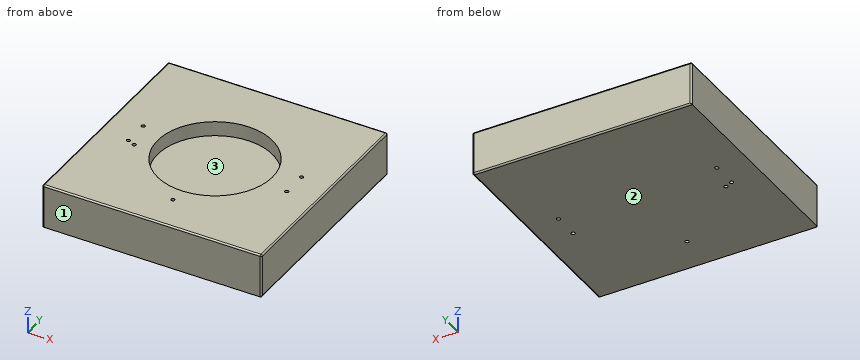
```python
from build123d import *

# Parameters (mm, degrees)
SKETCH1_W                   = 150
SKETCH1_H                   = 150
BOSS_EXTRUDE1_DEPTH         = 30
FILLET1_R                   = 1
SKETCH2_R                   = 39.25
CUT_EXTRUDE4_DEPTH          = 10
TAP_DRILL_FOR_M3X0_5_TAP2_D = 2.5
TAP_DRILL_FOR_M3X0_5_TAP3_D = 2.5
TAP_DRILL_FOR_M3X0_5_TAP5_D = 2.5


with BuildPart() as part:
    # Sketch1 → Boss-Extrude1 (new body)
    with BuildSketch(Plane.XY):
        Rectangle(SKETCH1_W, SKETCH1_H)
    extrude(amount=-BOSS_EXTRUDE1_DEPTH)

    # Fillet1
    fillet1_edges = [part.edges().sort_by_distance(p)[0] for p in [
        (0, 75, -30),
        (-75, 0, 0),
        (0, 75, 0),
        (75, 0, 0),
        (0, -75, 0),
        (-75, -75, -15),
        (-75, 75, -15),
        (75, 75, -15),
        (75, -75, -15),
        (75, 0, -30),
    ]]
    fillet(fillet1_edges, radius=FILLET1_R)

    # Sketch2 → Cut-Extrude4 (cut)
    with BuildSketch(Plane.XY):
        Circle(SKETCH2_R)
    extrude(amount=-CUT_EXTRUDE4_DEPTH, mode=Mode.SUBTRACT)

    # Tap Drill for M3x0.5 Tap2 (through all)
    with Locations(Plane.XY):
        with Locations((-54.190883488, -8.8), (-54.190883488, 8.8), (54.190883488, -8.8), (54.190883488, 8.8)):
            Hole(TAP_DRILL_FOR_M3X0_5_TAP2_D / 2)

    # Tap Drill for M3x0.5 Tap3 (through all)
    with Locations(Plane.XY):
        with Locations((-49, -11)):
            Hole(TAP_DRILL_FOR_M3X0_5_TAP3_D / 2)

    # Tap Drill for M3x0.5 Tap5 (through all)
    with Locations(Plane.XY):
        with Locations((-0.083892693, -49.999977478)):
            Hole(TAP_DRILL_FOR_M3X0_5_TAP5_D / 2)


solid = part.part
```
Input: part model. Units: mm. Frame: model coordinates. Face numbers are marked on the shaded views. Coordinates: 2 decimals unless noted, no trailing zeros. Loops run counter-clockwise (first coordinate to the right, second up) from the corner with the lowest first, then second, coordinate; pieces in that order, holes last. Notation, with made-up numbers: M 24,19 L 52,19 A34 cw 52,54 Z; hole C -14.5,34.5 d3. An arc over 180 degrees is marked long. Use a Markdown table: item, result. Add a question column.
1) Section B-B, the plane y = -34. Return the cut outline in (x, z).
2) Section A-A, the plane z = -3. Return the cut outline in (x, y), plus the area to 3 significant figures.
3) Line query: L1, parallel to X at y = 8.5, z = -20; L2, parallel to Y at x = 0, z = -6.25; L3, parallel to X at y = -12, z = -8.5. Output: solid intervals per line, ascending. Write a range as from..to.
4) Pin query (flat end, axial travel): P1, Ø2, axis at x = -0.08, y = -50, coming from the +Z side; P2, Ø3, axis at x = 54.19, y = 8.8, coming from the -Z side. Return the tip coordinate at first contact, or that it passes through.
5) Draft query along Y for the marked faces 1, 2 and 3. Return one class per face: +Y half, -Y half, draft (parallel to the pull), parting line (faces both ways), or undercut.
6) Section C-C, the plane y = 0. Return the cut outline in (x, z), plus the area to 3 significant figures.
Answer below:
| question | item | result |
|---|---|---|
| 1 | outline | M -75,-30 L 74,-30 A1 ccw 75,-29 L 75,-1 A1 ccw 74,0 L 19.61,0 L 19.61,-10 L -19.61,-10 L -19.61,0 L -74,0 A1 ccw -75,-1 Z |
| 2 | outline | M -75,-74 A1 ccw -74,-75 L 74,-75 A1 ccw 75,-74 L 75,74 A1 ccw 74,75 L -74,75 A1 ccw -75,74 Z; hole C -54.19,-8.8 d2.5; hole C -54.19,8.8 d2.5; hole C -49,-11 d2.5; hole C 0,0 d78.5; hole C -0.08,-50 d2.5; hole C 54.19,-8.8 d2.5; hole C 54.19,8.8 d2.5 |
| 2 | area | 17,600 mm2 |
| 3 | L1 | -75..-55.4, -52.98..52.98, 55.4..75 |
| 3 | L2 | -75..-51.25, -48.75..-39.25, 39.25..75 |
| 3 | L3 | -75..-49.75, -48.25..-37.37, 37.37..75 |
| 4 | P1 | through |
| 4 | P2 | z = -30 |
| 5 | face 1 | -Y half |
| 5 | face 2 | draft |
| 5 | face 3 | undercut |
| 6 | outline | M -75,-30 L 74,-30 A1 ccw 75,-29 L 75,-1 A1 ccw 74,0 L 39.25,0 L 39.25,-10 L -39.25,-10 L -39.25,0 L -74,0 A1 ccw -75,-1 Z |
| 6 | area | 3,710 mm2 |
